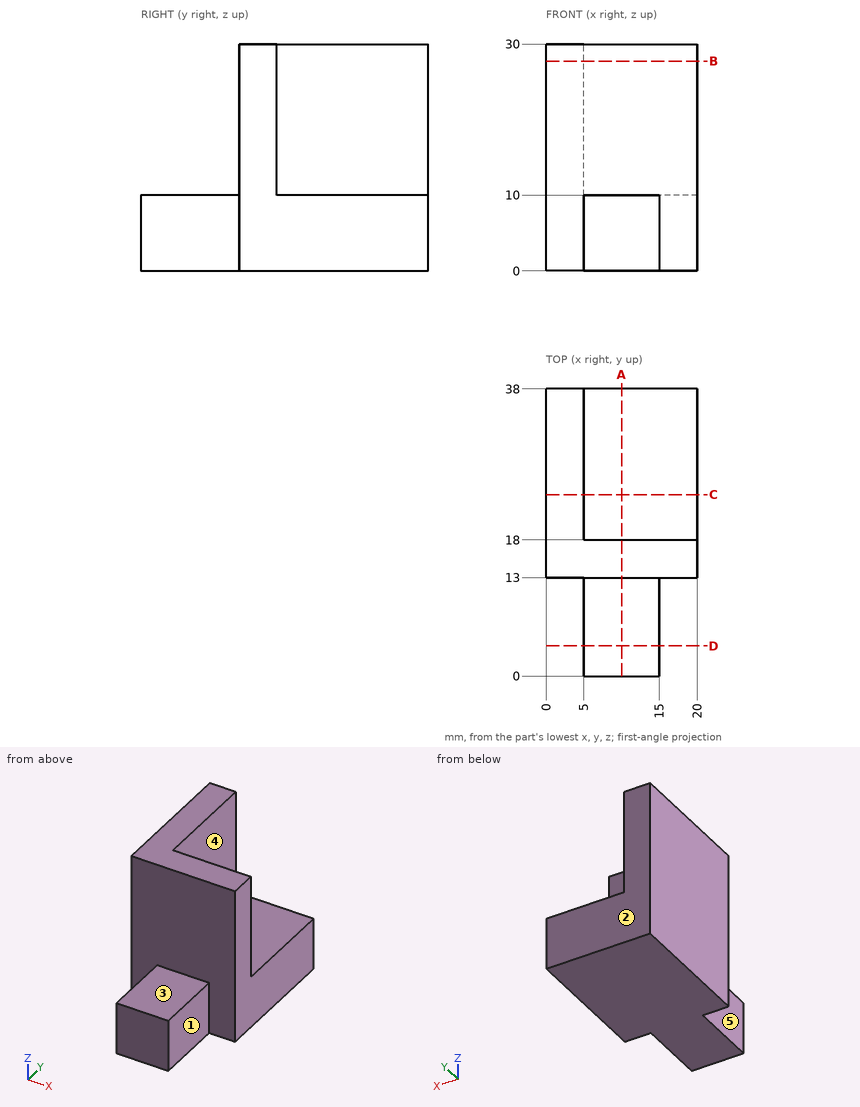
The figure shows three views and two pictorial views of one solid part (mm, origin at its lowest corner). Answer the questions. A direction names the side the tool comes from. Round coordinates to 2 decimals unless told otherwise and drop trailing zeros. Order: outer loops, then holes, each group sorted by start corner. A loop starts at its lowest first (then second) coordinate and runs counter-clockwise, first axis right, second up. Notation, with made-up numbers: (53, 30.5) -> (107, 30.5) arc R23 cw to (107, 61.5) -> close; hole circle Ø1 at (7.25, 26.5). An arc over 180 degrees is marked (long way). One line per item, written item: value.
Item 1: For the marked faces 1, 2, 3, 4 and 5, determine the directions among +Z, -Z, +X, -X, +Y, -Y from which every point of the face is accessible in a straight line to the end or side of a thin tool.
Taken from the geometry:
face 1: +Z, -Z, +X, -Y
face 2: +Z, -Z, +X, -X, +Y
face 3: +Z, +X, -X, -Y
face 4: +Z, +X, +Y
face 5: +Z, -Z, -X, -Y
Item 2: Find section C-C, the plane y = 24. Give the vertices of the cut face in (x, z).
Taken from the geometry:
outline: (0, 0) -> (20, 0) -> (20, 10) -> (5, 10) -> (5, 30) -> (0, 30) -> close
Item 3: Find section B-B, the plane z = 27.75. Give the vertices of the cut face in (x, y), then the cut area to 3 significant figures.
Taken from the geometry:
outline: (0, 13) -> (20, 13) -> (20, 18) -> (5, 18) -> (5, 38) -> (0, 38) -> close
area: 200 mm2
Item 4: Find section D-D, the plane y = 4. Give the vertices of the cut face in (x, z), then the cut area to 3 significant figures.
Taken from the geometry:
outline: (5, 0) -> (15, 0) -> (15, 10) -> (5, 10) -> close
area: 100 mm2
Item 5: Find section A-A, the plane x = 10. Give the vertices of the cut face in (y, z), then the cut area to 3 significant figures.
Taken from the geometry:
outline: (0, 0) -> (38, 0) -> (38, 10) -> (18, 10) -> (18, 30) -> (13, 30) -> (13, 10) -> (0, 10) -> close
area: 480 mm2
Item 6: Straight lines are drawn through the part: L1, parallel to Z at x = 10.5, y = 25.5; L2, parallel to Y at x = 15.5, z = 19.25; L3, parallel to X at y = 26, z = 27.75. For each, find the intervals that lie inside material, in ascending order.
Taken from the geometry:
L1: z = 0 to 10
L2: y = 13 to 18
L3: x = 0 to 5
Item 7: Given P1, Ø3, axis at y = 8, z = 3, coming from the -X side; P2, Ø4.5, axis at x = 16, z = 19.5, coming from the +Y side; P3, Ø5, axis at x = 12, y = 5, coming from the +Z side, each flat-ended and moving along its own axis, determine where each tip first touches the part or whether it passes through.
Taken from the geometry:
P1: stops at x = 5
P2: stops at y = 18
P3: stops at z = 10
